from build123d import *

# Parameters (mm, degrees)
SKETCH1_W                  = 80
SKETCH1_H                  = 12.65
BOSS_EXTRUDE1_DEPTH        = 6.325
M3_TAPPED_HOLE1_AT_2_COUNT = 2
M3_TAPPED_HOLE1_AT_2_PITCH = 15
M3_TAPPED_HOLE1_AT_3_COUNT = 2
M3_TAPPED_HOLE1_AT_3_PITCH = 55.5
M3_TAPPED_HOLE1_AT_4_COUNT = 2
M3_TAPPED_HOLE1_AT_4_PITCH = 70.5
SCALE1_SCALE               = 3


with BuildPart() as part:
    # Sketch1 → Boss-Extrude1 (new, symmetric)
    with BuildSketch(Plane(origin=(0, 0, 0), x_dir=(1, 0, 0), z_dir=(0, 1, 0))):
        Rectangle(SKETCH1_W, SKETCH1_H)
        with BuildLine():
            ThreePointArc((0, -3.241045356), (-8.575, 0), (0, 3.241045356))
            ThreePointArc((0, 3.241045356), (5.407411614, 4.583530299), (8.575, 0))
            ThreePointArc((8.575, 0), (5.407411614, -4.583530299), (0, -3.241045356))
        make_face(mode=Mode.SUBTRACT)
    extrude(amount=BOSS_EXTRUDE1_DEPTH, both=True)

    # Sketch5 → M3 Tapped Hole1 (revolve, cut)
    with BuildSketch(Plane(origin=(-35.25, 0, -6.325), x_dir=(0, 1, 0), z_dir=(1, 0, 0))):
        Polygon((0, 0), (0, 12.65), (1.75, 12.65), (1.25, 12.15), (1.25, 0.5), (1.75, 0), align=None)
    m3_tapped_hole1 = revolve(axis=Axis((-35.25, 0, -12.675), (0, 0, 1)), mode=Mode.SUBTRACT)

    # M3 Tapped Hole1 at 2: M3 Tapped Hole1 ×2
    with Locations(*[(i * M3_TAPPED_HOLE1_AT_2_PITCH, 0, 0) for i in range(1, M3_TAPPED_HOLE1_AT_2_COUNT)]):
        add(m3_tapped_hole1, mode=Mode.SUBTRACT)

    # M3 Tapped Hole1 at 3: M3 Tapped Hole1 ×2
    with Locations(*[(i * M3_TAPPED_HOLE1_AT_3_PITCH, 0, 0) for i in range(1, M3_TAPPED_HOLE1_AT_3_COUNT)]):
        add(m3_tapped_hole1, mode=Mode.SUBTRACT)

    # M3 Tapped Hole1 at 4: M3 Tapped Hole1 ×2
    with Locations(*[(i * M3_TAPPED_HOLE1_AT_4_PITCH, 0, 0) for i in range(1, M3_TAPPED_HOLE1_AT_4_COUNT)]):
        add(m3_tapped_hole1, mode=Mode.SUBTRACT)


with BuildPart() as part_1:
    # Scale1: scaled about (0, 0, 0)
    add(part.part.scale(SCALE1_SCALE))


solid = part_1.part
Read the model definition and answer for the solid it produces. Units are mm, in the model's axes. Round coordinates to 2 decimals unless told otherwise and drop trailing zeros. Write each loop counter-clockwise with the first axis right and the second up, starting at its lowest first coordinate (ties: lowest second). Pieces come first, ordered by that corner, then holes. Notation, with made-up numbers: (48.5, 33) - (82.5, 33) arc R22 ccw to (82.5, 71) - close; hole circle Ø6 at (-27.75, 60.25). An arc over 180 degrees is marked (long way). One line per question, with ' | ' between items. Start each with the question number.
1. Section A-A (z = 3.5) is taken. Determine the outline of the cut face in (x, y) (3 decimals), and give its area (3 significant figures).
2. Section B-B (x = -105.75) is taken. Determine the outline of the cut face in (y, z) (3 decimals), and give its area (3 significant figures).
3. Section C-C (z = 12.5) is taken. Determine the outline of the cut face in (x, y) (3 decimals), and give its area (3 significant figures).
4. Find the intervals of material crossed by probe 1 along Y at (x, z) = (-105.75, 0) (3 decimals); probe 2 along X at (y, z) = (7, 0.5); probe 3 along X at (y, z) = (-16.5, 11.5), in increasing order. Write a range as [from, to].
5. Each of these flat-tipped pins is pushed along its axis until it touches: pin 1 (8.5 mm diameter, centred on x = 60.75, y = 0, fed in from +Z) (3 decimals); pin 2 (12 mm diameter, centred on x = -105.75, y = 0, fed in from -Z) (3 decimals); pin 3 (10 mm diameter, centred on x = -60.75, y = 0, fed in from +Z) (3 decimals). Where does it stop, or does it pass through?
6. Section D-D (y = 0) is taken. Give the number of separate pieces and of enclosed holes in the cut face, and give its area (3 significant figures).
7. For a pull along Z with two mould halves and no side action, classify faces 1 (the face through (-61.9, 3.7, -17.6)), 2 (the face through (120, 0, 0)), 3 (the face through (-25.717, -0.266, 0.498)), 4 (the face through (25.717, 0.266, -0.498)) as +Z half, -Z half, draft (parallel to the pull), parting line (faces both ways), or undercut.
Filled in:
1) outline: (-120, -18.975) - (-25.302, -18.975) - (-25.302, 18.975) - (-120, 18.975) - close; (25.302, -18.975) - (120, -18.975) - (120, 18.975) - (25.302, 18.975) - close; hole circle Ø7.5 at (-105.75, 0); hole circle Ø7.5 at (-60.75, 0); hole circle Ø7.5 at (60.75, 0); hole circle Ø7.5 at (105.75, 0) | area: 7,010 mm²
2) outline: (-18.975, -18.975) - (-5.25, -18.975) - (-3.75, -17.475) - (-3.75, 17.475) - (-5.25, 18.975) - (-18.975, 18.975) - close; (3.75, -17.475) - (5.25, -18.975) - (18.975, -18.975) - (18.975, 18.975) - (5.25, 18.975) - (3.75, 17.475) - close | area: 1,150 mm²
3) outline: (-120, -18.975) - (-18.761, -18.975) - (-18.761, 18.975) - (-120, 18.975) - close; (-3.289, -18.975) - (3.289, -18.975) - (3.289, 18.975) - (-3.289, 18.975) - close; (18.761, -18.975) - (120, -18.975) - (120, 18.975) - (18.761, 18.975) - close; hole circle Ø7.5 at (-105.75, 0); hole circle Ø7.5 at (-60.75, 0); hole circle Ø7.5 at (60.75, 0); hole circle Ø7.5 at (105.75, 0) | area: 7,760 mm²
4) probe 1: [-18.975, -3.75], [3.75, 18.975] | probe 2: [-120, -25.72], [25.72, 120] | probe 3: [-120, -20.18], [-1.87, 1.87], [20.18, 120]
5) pin 1: z = 17.975 | pin 2: z = -18.975 | pin 3: z = 18.725
6) separate pieces: 5 | enclosed holes: 1 | area: 6,690 mm²
7) face 1: -Z half | face 2: draft | face 3: undercut | face 4: undercut
